```python
from build123d import *

# Parameters (mm, degrees)
CIRPATTERN1_COUNT = 16
CIRPATTERN2_COUNT = 8
CIRPATTERN3_COUNT = 2


with BuildPart() as part:
    # Sketch1 → Revolve1 (revolve)
    with BuildSketch(Plane.XY):
        Polygon((-76.2, 19.05), (-76.2, 0), (-42.8625, 0), (-25.4, 15.875), (-19.05, 15.875), (-19.05, 60.325), (-25.4, 60.325), (-25.4, 73.025), (-50.8, 73.025), (-50.8, 19.05), align=None)
    revolve(axis=Axis((0, 0, 0), (0, 1, 0)))

    # Sketch5 → 5_16 _0.3125_ Diameter Hole1 (revolve, cut)
    with BuildSketch(Plane(origin=(-69.85, 19.05, 0), x_dir=(0, 0, 1), z_dir=(1, 0, 0))):
        Polygon((0, 0), (0, 40.484665582), (3.96875, 38.1), (3.96875, 0), align=None)
    f_5_16_0_3125_diameter_hole1 = revolve(axis=Axis((-69.85, 25.4, 0), (0, -1, 0)), mode=Mode.SUBTRACT)

    # CirPattern1: 5_16 _0.3125_ Diameter Hole1 ×16 about axis
    cirpattern1_axis = Axis((0, 0, 0), (0, 1, 0))
    for i in range(1, CIRPATTERN1_COUNT):
        add(f_5_16_0_3125_diameter_hole1.rotate(cirpattern1_axis, i * 360 / CIRPATTERN1_COUNT), mode=Mode.SUBTRACT)

    # Sketch7 → 5_16 _0.3125_ Diameter Hole2 (revolve, cut)
    with BuildSketch(Plane(origin=(44.45, 73.025, 0), x_dir=(0, 0, 1), z_dir=(1, 0, 0))):
        Polygon((0, 0), (0, 27.784665582), (3.96875, 25.4), (3.96875, 0), align=None)
    f_5_16_0_3125_diameter_hole2 = revolve(axis=Axis((44.45, 79.375, 0), (0, -1, 0)), mode=Mode.SUBTRACT)

    # CirPattern2: 5_16 _0.3125_ Diameter Hole2 ×8 about axis
    cirpattern2_axis = Axis((0, 0, 0), (0, 1, 0))
    for i in range(1, CIRPATTERN2_COUNT):
        add(f_5_16_0_3125_diameter_hole2.rotate(cirpattern2_axis, i * 360 / CIRPATTERN2_COUNT), mode=Mode.SUBTRACT)

    # Sketch9 → 1_4 NPT Tapped Hole1 (revolve, cut)
    with BuildSketch(Plane(origin=(46.933080252, 50.8, -19.440318364), x_dir=(-0.382683432, 0, -0.923879533), z_dir=(0, 1, 0))):
        Polygon((0, 0), (0, 41.442347279), (5.5626, 38.1), (5.5626, 9.906), (5.943685794, 9.906), (6.2402847, 0), align=None)
    revolve(axis=Axis((52.799715283, 50.8, -21.87035816), (-0.923879533, 0, 0.382683432)), mode=Mode.SUBTRACT)

    # Sketch13 → Tap Drill for 1_2-13 Tap1 (revolve, cut)
    with BuildSketch(Plane(origin=(-14.580238773, 73.025, -35.199810189), x_dir=(0, 0, 1), z_dir=(1, 0, 0))):
        Polygon((0, 0), (0, 66.719489309), (5.35813, 63.5), (5.35813, 0), align=None)
    tap_drill_for_1_2_13_tap1 = revolve(axis=Axis((-14.580238773, 79.375, -35.199810189), (0, -1, 0)), mode=Mode.SUBTRACT)

    # CirPattern3: Tap Drill for 1_2-13 Tap1 ×2 about axis
    cirpattern3_axis = Axis((0, 0, 0), (0, 1, 0))
    for i in range(1, CIRPATTERN3_COUNT):
        add(tap_drill_for_1_2_13_tap1.rotate(cirpattern3_axis, i * 360 / CIRPATTERN3_COUNT), mode=Mode.SUBTRACT)


solid = part.part
```
Geometry: final body of the model. Coordinates: model frame, mm. A direction names the side the tool comes from. Coordinates: 2 decimals unless noted, no trailing zeros. Order: outer loops, then holes, each group sorted by start corner. A loop starts at its lowest first (then second) coordinate and runs counter-clockwise, first axis right, second up. Notation, with made-up numbers: (-20.5, -38) -> (15.5, -38) arc R19 cw to (15.5, -12) -> close; hole circle Ø3 at (-20.5, 54). An arc over 180 degrees is marked (long way). Answer in a Markdown table with one row per item.
Item 1: Ray query, L1, parallel to Z at x = 0, y = 60.75; L2, parallel to Z at x = 1.5, y = 66; L3, parallel to Z at x = 16.5, y = 21.5. Return the intervals inside material, ascending.
Return value:
| item | result |
|---|---|
| L1 | z = -50.8 to -48.42, -40.48 to -25.4, 25.4 to 40.48, 48.42 to 50.8 |
| L2 | z = -50.78 to -48.12, -40.78 to -25.36, 25.36 to 40.78, 48.12 to 50.78 |
| L3 | z = -48.05 to -9.52, 9.52 to 30.2, 40.2 to 48.05 |
Item 2: Draft query along X for faces 1 (the cylindrical face through (-68.44, 9.66, -26.04)), 2 (the flat face through (-33, 0, -33)), 3 (the cylindrical face through (11.012, 45.66, -49.592)). Return one class per face: released by +X, released by -X, zero draft, split by the parting line, or undercut.
Return value:
| item | result |
|---|---|
| face 1 | undercut |
| face 2 | zero draft |
| face 3 | split by the parting line |
Item 3: Contact query for flat-ended pins moving along their axis: P1, Ø8.5, axis at x = 14.58, z = 35.2, coming from the +Y side; P2, Ø10, axis at y = 51.5, z = -1.5, coming from the -X side; P3, Ø5, axis at y = 10, z = 12, coming from the -X side; P4, Ø7, axis at x = 64.53, z = -26.73, coming from the -Y side. Output: stop coordinate, or through.
Return value:
| item | result |
|---|---|
| P1 | stops at y = 8.86 |
| P2 | stops at x = -50.8 |
| P3 | stops at x = -75.61 |
| P4 | passes through |
Item 4: Access query for faces 4 (the cylindrical face through (-65.976, 9.658, -0.86)), 5 (the cylindrical face through (0.86, 60.503, 48.324)). Directions: +Z, -Z, +X, -X, +Y, -Y. A direction counts if a zero-diameter tool reaches every point of the face in a straight line with its end or side. Return the directions, or none.
Return value:
| item | result |
|---|---|
| face 4 | +Y, -Y |
| face 5 | +Y |
Item 5: Section A-A on y = 23. Output: boundary loops of the cut face in (x, z), plus the area to 3 significant figures.
Return value:
| item | result |
|---|---|
| outline | circle Ø101.6 at (0, 0); hole circle Ø10.72 at (-14.58, -35.2); hole circle Ø38.1 at (0, 0); hole circle Ø10.72 at (14.58, 35.2) |
| area | 6,790 mm² |
